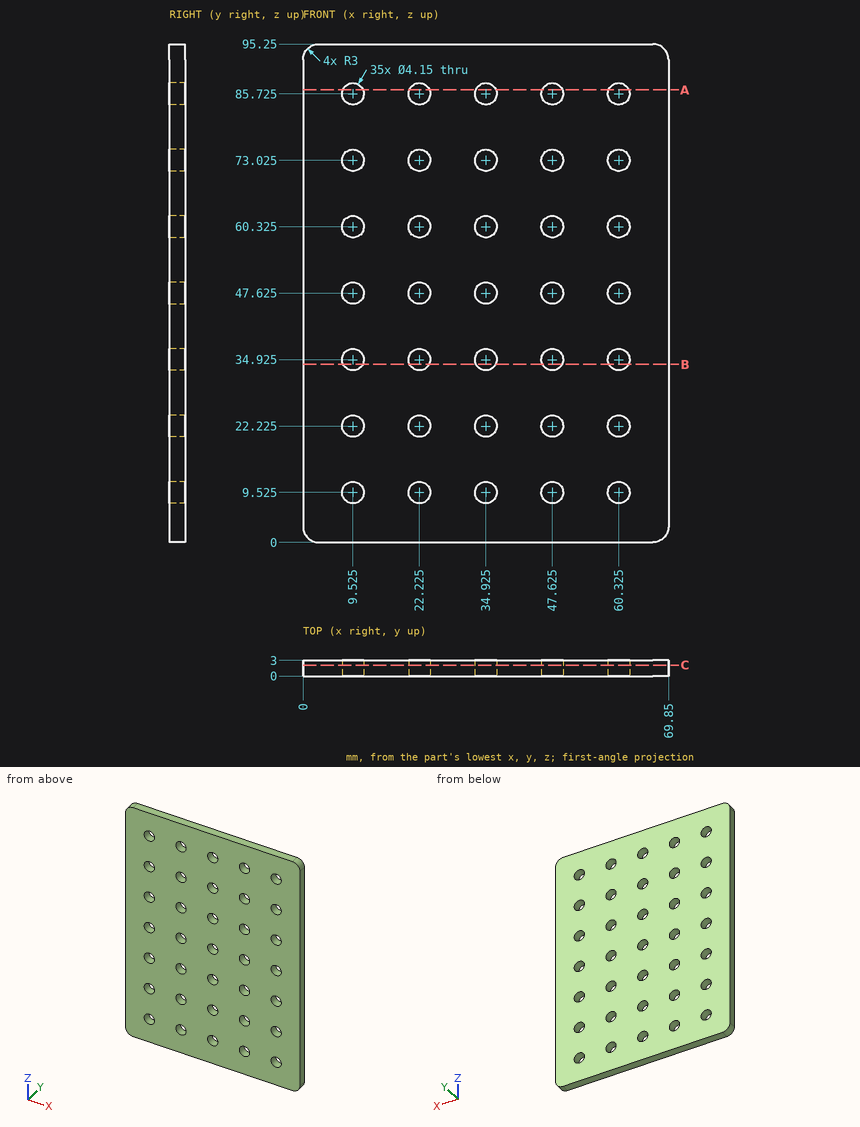
Job drawing, mm, ordinate dimensions from the low corner. One solid piece. Round coordinates to 2 decimals unless told otherwise and drop trailing zeros. Loops run counter-clockwise (first coordinate to the right, second up) from the corner with the lowest first, then second, coordinate; pieces in that order, holes last. Notation, with made-up numbers: (-22.5, 35) -> (11.5, 35) arc R16 cw to (11.5, 42) -> close; hole circle Ø4 at (20, 65). An arc over 180 degrees is marked (long way). Use a Markdown table: item, result.
1) Cut at B-B, the plane z = 34. List the corners of the cut face in (x, y), and give its area (3 significant figures).
The answers:
| item | result |
|---|---|
| outline | (0, 0) -> (7.67, 0) -> (7.67, 3) -> (0, 3) -> close; (11.38, 0) -> (20.37, 0) -> (20.37, 3) -> (11.38, 3) -> close; (24.08, 0) -> (33.07, 0) -> (33.07, 3) -> (24.08, 3) -> close; (36.78, 0) -> (45.77, 0) -> (45.77, 3) -> (36.78, 3) -> close; (49.48, 0) -> (58.47, 0) -> (58.47, 3) -> (49.48, 3) -> close; (62.18, 0) -> (69.85, 0) -> (69.85, 3) -> (62.18, 3) -> close |
| area | 154 mm2 |
2) Probe line 1 (X direction, y = 1.4, z = 35); line 2 (X direction, y = 2.55, z = 8.5). List the from-to ranges inside material, lowest first. Write a range as [from, to].
The answers:
| item | result |
|---|---|
| line 1 | x = [0, 7.45], [11.6, 20.15], [24.3, 32.85], [37, 45.55], [49.7, 58.25], [62.4, 69.85] |
| line 2 | x = [0, 7.72], [11.33, 20.42], [24.03, 33.12], [36.73, 45.82], [49.43, 58.52], [62.13, 69.85] |
3) Drop a flat-ended pin along its axis: pin 1 Ø5 at (x, z) = (34.925, 60.325) entering from +Y. Give the stop position or say it passes through.
The answers:
| item | result |
|---|---|
| pin 1 | stops at y = 3 |
4) Cut at A-A, the plane z = 86.5. List the corners of the cut face in (x, y), and give its area (3 significant figures).
The answers:
| item | result |
|---|---|
| outline | (0, 0) -> (7.6, 0) -> (7.6, 3) -> (0, 3) -> close; (11.45, 0) -> (20.3, 0) -> (20.3, 3) -> (11.45, 3) -> close; (24.15, 0) -> (33, 0) -> (33, 3) -> (24.15, 3) -> close; (36.85, 0) -> (45.7, 0) -> (45.7, 3) -> (36.85, 3) -> close; (49.55, 0) -> (58.4, 0) -> (58.4, 3) -> (49.55, 3) -> close; (62.25, 0) -> (69.85, 0) -> (69.85, 3) -> (62.25, 3) -> close |
| area | 152 mm2 |
5) Cut at C-C, the plane y = 2.1. State how many separate pieces and enclosed holes the cut face has, and give its area (3 significant figures).
The answers:
| item | result |
|---|---|
| separate pieces | 1 |
| enclosed holes | 35 |
| area | 6,170 mm2 |
